Autodesk Inventor part; units mm, degrees
ref_plane "YZ Plane" through (0, 0, 0) normal (1, 0, 0) x (0, 1, 0)
ref_plane "XZ Plane" through (0, 0, 0) normal (0, 1, 0) x (-1, 0, 0)
ref_plane "XY Plane" through (0, 0, 0) normal (0, 0, 1) x (1, 0, 0)
sketch "Sketch1" plane through (0, 0, 0) normal (0, 0, 1) x (1, 0, 0)
  line L0 (0, 0) -> (12.446, 0)
  line L1 (12.446, 0) -> (12.446, 5.588)
  line L2 (12.446, 5.588) -> (0, 5.588)
  line L3 (0, 5.588) -> (0, 0)
  line L4 (0, 5.588) -> (19.05, 5.588)
  line L5 (19.05, 5.588) -> (19.05, 9.525)
  line L6 (15.875, 12.7) -> (0, 12.7)
  line L7 (0, 12.7) -> (0, 5.588)
  arc A0 (19.05, 9.525) -> (15.875, 12.7) centre (15.875, 9.525) ccw
  dimension "d0" = 12.446
  dimension "d1" = 5.588
  dimension "d2" = 19.05
  dimension "d3" = 12.7
  dimension "d4" = 3.175
revolve "Revolution1" add sketch "Sketch1" angle 360 about axis through (0, 5.588, 0) along (0, -1, 0)
chamfer "Chamfer1" distance 1.5875 angle 45 1 edges at (-12.446, 0, 0)
properties part number "2016.06.10 ps Hamamatsu PMT Adapter bung cover"
Design review of the part built by this model. Coordinates are the model's own, in mm. A direction names the side the tool comes from. Coordinates: 2 decimals unless noted, no trailing zeros. Order: outer loops, then holes, each group sorted by start corner. A loop starts at its lowest first (then second) coordinate and runs counter-clockwise, first axis right, second up. Notation, with made-up numbers: (15, 5) -> (24, 5) arc R18 ccw to (24, 13) -> close; hole circle Ø9 at (-5.5, 65). An arc over 180 degrees is marked (long way). One line per item, written item: value. Start each with the question number.
Q1. Tool access review of faces 1 (the cylindrical face through (-2.7, 3.62, 12.15)), 2 (the flat face through (0, 0, 0)): name each direction out of +Z, -Z, +X, -X, +Y, -Y from which nothing blocks a thin tool from reaching the whole face with its end or side.
Q2. Take a section at C-C, the plane y = 4.75. State the section outline as (x, z) points, then the cut area to 3 significant figures.
Q3. Insertion check: pin 1 Ø3 at (y, z) = (8.5, 13.5) entering from -X; pin 2 Ø1 at (y, z) = (8, -12) entering from +X; pin 3 Ø1 at (x, y) = (10, 9) entering from -Z. Each pin has a flat end and moves straight along its axis. Give the tip position at first contact, or say it passes through.
Q4. Take a section at D-D, the plane y = 8. State the section outline as (x, z) points, then the cut area to 3 significant figures.
Q5. For probe 1 along Y at (x, z) = (-2.5, -15); probe 2 along X at (y, z) = (11.25, 14); probe 3 along X at (y, z) = (4.25, 10.5), list the stretches that pass through material, from the lowest coordinate up.
Values follow:
1. face 1: -Y
1. face 2: +Z, -Z, +X, -X, -Y
2. outline: circle Ø24.89 at (0, 0)
2. area: 487 mm2
3. pin 1: stops at x = -14.8
3. pin 2: stops at x = 15.19
3. pin 3: stops at z = -16.51
4. outline: circle Ø38.1 at (0, 0)
4. area: 1,140 mm2
5. probe 1: y = 5.59 to 12.7
5. probe 2: x = -12.16 to 12.16
5. probe 3: x = -6.68 to 6.68
